Part print with two shaded views. Sizes in mm from the minimum x, y, z corner. A direction names the side the tool comes from. Round coordinates to 2 decimals unless told otherwise and drop trailing zeros. Write each loop counter-clockwise with the first axis right and the second up, starting at its lowest first coordinate (ties: lowest second). Pieces come first, ordered by that corner, then holes. Notation, with made-up numbers: (88, 18.5) -> (97, 18.5) arc R18 ccw to (97, 39.5) -> close; hole circle Ø9 at (-1, 40.25). An arc over 180 degrees is marked (long way). Answer as CSV lines item,"result".
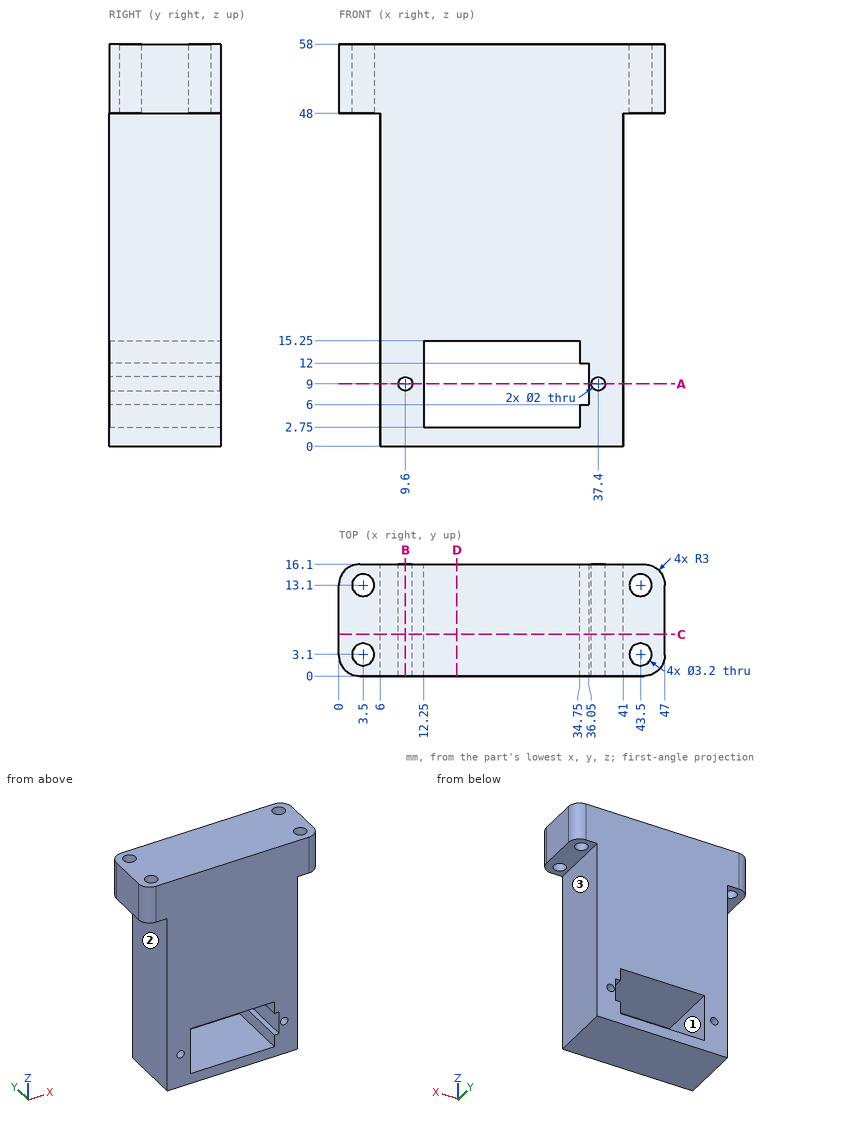
1. Probe line 1 along X through (y, z) = (10, 9); line 2 along Y through (x, z) = (3.5, 55.5); line 3 along X through (y, z) = (9.25, 6.5). List the from-to ranges inside material, lowest first.
Results found:
line 1,"x = 6 to 8.6, 10.6 to 12.25, 36.05 to 36.4, 38.4 to 41"
line 2,"y = 0 to 1.5, 4.7 to 11.5, 14.7 to 16.1"
line 3,"x = 6 to 12.25, 36.05 to 41"
2. Which spindle directions (+Z, -Z, +X, -X, +Y, -Y) get a long thin tool onto all of the face, cutting with end or side? Do the marked faces 1, 2 and 3. Say none if no direction does.
Results found:
face 1,"+Y, -Y"
face 2,"-Z, -X, +Y, -Y"
face 3,"-Z, +X, +Y, -Y"
3. Drop flat-ended pins along their axis: pin 1 Ø1.5 at (x, y) = (23.5, 9.5) entering from -Z; pin 2 Ø3.5 at (x, y) = (3.5, 3.1) entering from -Z; pin 3 Ø1.5 at (y, z) = (8, 44.5) entering from -X. Give the stop position or say it passes through.
Results found:
pin 1,"stops at z = 0"
pin 2,"stops at z = 48"
pin 3,"stops at x = 6"
4. Cut at D-D, the plane x = 17. Write the cut outline in (y, z).
Results found:
outline,"(0, 0) -> (16.1, 0) -> (16.1, 2.75) -> (0, 2.75) -> close; (0, 15.25) -> (16.1, 15.25) -> (16.1, 58) -> (0, 58) -> close"
5. Cut at C-C, the plane y = 6. Write the cut outline in (x, z).
Results found:
outline,"(0, 48) -> (6, 48) -> (6, 0) -> (41, 0) -> (41, 48) -> (47, 48) -> (47, 58) -> (0, 58) -> close; hole circle Ø2 at (9.6, 9); hole (12.25, 2.75) -> (34.75, 2.75) -> (34.75, 6) -> (36.05, 6) -> (36.05, 12) -> (34.75, 12) -> (34.75, 15.25) -> (12.25, 15.25) -> close; hole circle Ø2 at (37.4, 9)"
6. Cut at B-B, the plane x = 9.6. Write the cut outline in (y, z).
Results found:
outline,"(0, 0) -> (16.1, 0) -> (16.1, 8) -> (0, 8) -> close; (0, 10) -> (16.1, 10) -> (16.1, 58) -> (0, 58) -> close"
7. Cut at A-A, the plane z = 9. Write the cut outline in (x, y).
Results found:
outline,"(6, 0) -> (8.6, 0) -> (8.6, 16.1) -> (6, 16.1) -> close; (10.6, 0) -> (12.25, 0) -> (12.25, 16.1) -> (10.6, 16.1) -> close; (36.05, 0) -> (36.4, 0) -> (36.4, 16.1) -> (36.05, 16.1) -> close; (38.4, 0) -> (41, 0) -> (41, 16.1) -> (38.4, 16.1) -> close"
